```python
from build123d import *

# Parameters (mm, degrees)
SKETCH1_W                      = 104.072
SKETCH1_H                      = 82.6
BASE_FLANGE2_DEPTH             = 1
EDGE_FLANGE1_STRIP_W           = 6
EDGE_FLANGE1_STRIP_H           = 1
EDGE_FLANGE1_STRIP_CUT_DEPTH   = 82.6
EDGE_FLANGE1_STRIP_2_W         = 6
EDGE_FLANGE1_STRIP_2_H         = 1
EDGE_FLANGE1_STRIP_CUT_2_DEPTH = 82.6
EDGE_FLANGE1_DEPTH             = 82.6
EDGE_FLANGE1_BEND_DEPTH        = 82.6
SKETCH16_W                     = 66.6
SKETCH16_H                     = 7
CUT_EXTRUDE1_DEPTH             = 134.051648558
FILLET1_R                      = 1
SKETCH17_R                     = 2
CUT_EXTRUDE2_DEPTH             = 134.051648558


# Sheet-metal steps are written as plain solids
with BuildPart() as part:
    # Sketch1 → Base-Flange2 (new body)
    with BuildSketch(Plane(origin=(0, 0, 0), x_dir=(1, 0, 0), z_dir=(0, 1, 0))):
        with Locations((52.036, 41.3)):
            Rectangle(SKETCH1_W, SKETCH1_H)
    extrude(amount=-BASE_FLANGE2_DEPTH)

    # Edge-Flange1 strip (across the edge) → Edge-Flange1 strip cut (cut)
    with BuildSketch(Plane(origin=(104.072, 0, 0), x_dir=(-1, 0, 0), z_dir=(0, 0, -1))):
        with Locations((-1, -0.5)):
            Rectangle(EDGE_FLANGE1_STRIP_W, EDGE_FLANGE1_STRIP_H)
    extrude(amount=EDGE_FLANGE1_STRIP_CUT_DEPTH, mode=Mode.SUBTRACT)

    # Edge-Flange1 strip 2 (across the edge) → Edge-Flange1 strip cut 2 (cut)
    with BuildSketch(Plane.XY.offset(-82.6)):
        with Locations((-1, -0.5)):
            Rectangle(EDGE_FLANGE1_STRIP_2_W, EDGE_FLANGE1_STRIP_2_H)
    extrude(amount=EDGE_FLANGE1_STRIP_CUT_2_DEPTH, mode=Mode.SUBTRACT)

    # Edge-Flange1 section (across the edge) → Edge-Flange1 (add)
    with BuildSketch(Plane(origin=(104.072, 0, 0), x_dir=(-1, 0, 0), z_dir=(0, 0, -1))):
        with BuildLine():
            Line((0, 1), (0, 7))
            Line((0, 7), (1, 7))
            Line((1, 7), (1, 1))
            ThreePointArc((1, 1), (1.292893219, 0.292893219), (2, 0))
            Line((2, 0), (2, -1))
            ThreePointArc((2, -1), (0.585786438, -0.414213562), (0, 1))
        make_face()
    extrude(amount=EDGE_FLANGE1_DEPTH)

    # Edge-Flange1 section 2 (across the edge) → Edge-Flange1 bend (add)
    with BuildSketch(Plane.XY.offset(-82.6)):
        with BuildLine():
            Line((0, 1), (0, 7))
            Line((0, 7), (1, 7))
            Line((1, 7), (1, 1))
            ThreePointArc((1, 1), (1.292893219, 0.292893219), (2, 0))
            Line((2, 0), (2, -1))
            ThreePointArc((2, -1), (0.585786438, -0.414213562), (0, 1))
        make_face()
    extrude(amount=EDGE_FLANGE1_BEND_DEPTH)

    # Sketch16 → Cut-Extrude1 (cut, through all)
    with BuildSketch(Plane(origin=(104.072, 0, 0), x_dir=(0, 0, -1), z_dir=(1, 0, 0))):
        with Locations((41.3, 4.5)):
            Rectangle(SKETCH16_W, SKETCH16_H)
    extrude(amount=-CUT_EXTRUDE1_DEPTH, mode=Mode.SUBTRACT)

    # Fillet1
    fillet1_edges = [part.edges().sort_by_distance(p)[0] for p in [
        (103.572, 7, 0),
        (103.572, 7, -82.6),
        (0.5, 7, -82.6),
        (0.5, 7, 0),
        (0.5, 7, -74.6),
        (0.5, 7, -8),
        (103.572, 7, -8),
        (103.572, 7, -74.6),
    ]]
    fillet(fillet1_edges, radius=FILLET1_R)

    # Sketch17 → Cut-Extrude2 (cut, through all)
    with BuildSketch(Plane(origin=(104.072, 0, 0), x_dir=(0, 0, -1), z_dir=(1, 0, 0))):
        with Locations(Location((4, 4, 0), (0, 0, 90))):
            Circle(SKETCH17_R)
        with Locations(Location((78.6, 4, 0), (0, 0, 90))):
            Circle(SKETCH17_R)
    extrude(amount=-CUT_EXTRUDE2_DEPTH, mode=Mode.SUBTRACT)


solid = part.part
```
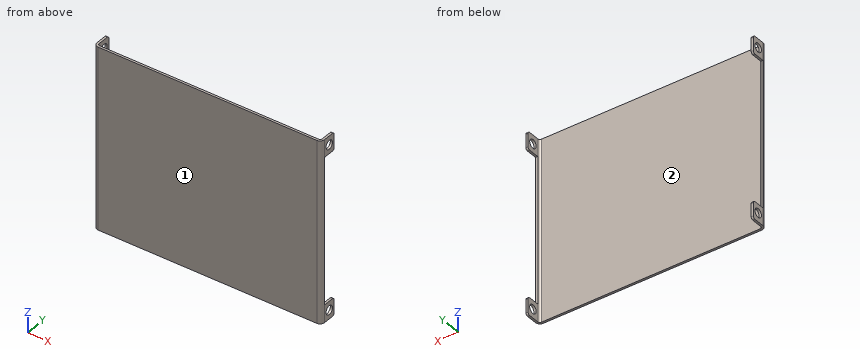
Source: CAD feature listing. Evaluate the final solid. Frame: model axes, mm. Face numbers are marked on the shaded views. A direction names the side the tool comes from. Round coordinates to 2 decimals unless told otherwise and drop trailing zeros. Loops run counter-clockwise (first coordinate to the right, second up) from the corner with the lowest first, then second, coordinate; pieces in that order, holes last.
1. Contact query for flat-ended pins moving along their axis: pin 1 (3.5 mm diameter, centred on y = 4, z = -4, fed in from +X); pin 2 (8 mm diameter, centred on x = 55.5, z = -26, fed in from +Y); pin 3 (0.8 mm diameter, centred on x = 0.5, z = -31, fed in from +Y). Output: stop coordinate, or through.
2. Ray query, L1, parallel to Z at x = 103.6, y = 4; L2, parallel to Y at x = 67, z = -34.5; L3, parallel to X at y = 0.25, z = -5. Return the intervals inside material, ascending.
3. Section query A-A on y = 4. Give the number of separate pieces and of enclosed holes in the cut face, and give its area (3 significant figures).
4. Section query B-B on z = -37.5. Output: boundary loops of the cut face in (x, y).
5. Section query C-C on z = -4. Output: boundary loops of the cut face in (x, y), and give its area (3 significant figures).
6. Access query for the marked faces 1 and 2. Directions: +Z, -Z, +X, -X, +Y, -Y. A direction counts if a zero-diameter tool reaches every point of the face in a straight line with its end or side. Return the directions, or none.
7. Section query D-D on x = 83.5. Output: boundary loops of the cut face in (y, z).
Answers below:
1. pin 1: passes through
1. pin 2: stops at y = 0
1. pin 3: stops at y = 1
2. L1: z = -82.6 to -80.6, -76.6 to -74.6, -8 to -6, -2 to 0
2. L2: y = -1 to 0
2. L3: x = 0.15 to 1.34, 102.73 to 103.93
3. separate pieces: 8
3. enclosed holes: 0
3. area: 16.0 mm2
4. outline: (0, 1) arc R2 ccw to (2, -1) - (102.07, -1) arc R2 ccw to (104.07, 1) - (103.07, 1) arc R1 cw to (102.07, 0) - (2, 0) arc R1 cw to (1, 1) - close
5. outline: (0, 1) arc R2 ccw to (2, -1) - (102.07, -1) arc R2 ccw to (104.07, 1) - (104.07, 2) - (103.07, 2) - (103.07, 1) arc R1 cw to (102.07, 0) - (2, 0) arc R1 cw to (1, 1) - (1, 2) - (0, 2) - close; (0, 6) - (1, 6) - (1, 7) - (0, 7) - close; (103.07, 6) - (104.07, 6) - (104.07, 7) - (103.07, 7) - close
5. area: 109 mm2
6. face 1: +Z, -Z, +X, -X, -Y
6. face 2: +Z, -Z, +Y
7. outline: (-1, -82.6) - (0, -82.6) - (0, 0) - (-1, 0) - close
